Verification items for the finished model (mm, model axes). Face numbers are marked on the shaded views. A direction names the side the tool comes from. Coordinates: 2 decimals unless noted, no trailing zeros. Write each loop counter-clockwise with the first axis right and the second up, starting at its lowest first coordinate (ties: lowest second). Pieces come first, ordered by that corner, then holes. Notation, with made-up numbers: (-38, 71.25) -> (3, 71.25) arc R23 ccw to (3, 103.25) -> close; hole circle Ø6 at (33, 22). An arc over 180 degrees is marked (long way). Answer in a Markdown table with one row per item.
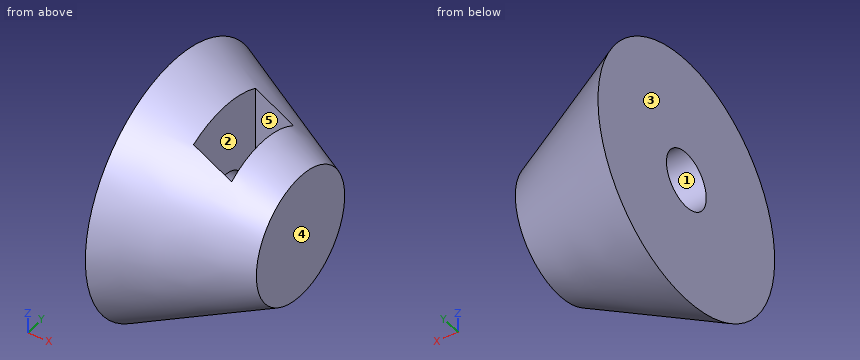
Autodesk Inventor part; units mm, degrees
ref_plane "Work Plane1" through (7, 0, 0) normal (1, 0, 0) x (0, 1, 0)
ref_plane "XZ Plane" through (0, 0, 0) normal (0, 1, 0) x (-1, 0, 0)
ref_plane "XY Plane" through (0, 0, 0) normal (0, 0, 1) x (1, 0, 0)
ref_plane "Work Plane1" through (7, 0, 0) normal (1, 0, 0) x (0, 1, 0)
sketch "Sketch1" plane through (0, 0, 0) normal (0, 1, 0) x (-1, 0, 0)
  line L0 (0, 0) -> (-10, 0)
  line L1 (0, 0) -> (0, -10)
  line L2 (-10, 0) -> (-10, -5)
  line L3 (-10, -5) -> (0, -10)
  dimension "d0" = 10
  dimension "d1" = 10
  dimension "d2" = 5
revolve "Revolution1" add sketch "Sketch1" angle 360 about axis through (0, 0, 0) along (1, 0, 0)
sketch "Sketch2" plane through (7, 0, 0) normal (1, 0, 0) x (0, 1, 0)
  circle A0 centre (0, 0) radius 2.25
  dimension "d5" = 4.5
extrude "Extrusion1" cut sketch "Sketch2" along normal blind 2 and the other way blind 10
sketch "Sketch3" plane through (7, 0, 0) normal (1, 0, 0) x (0, 1, 0)
  line L0 (-3.5, 3.5) -> (3.5, 3.5)
  line L1 (3.5, 3.5) -> (3.5, -3.5)
  line L2 (3.5, -3.5) -> (-3.5, -3.5)
  line L3 (-3.5, -3.5) -> (-3.5, 3.5)
  line L4 (-3.5, 3.5) -> (3.5, -3.5) construction
  line L5 (3.5, 3.5) -> (-3.5, -3.5) construction
  line L6 (-3.5, 3.5) -> (3.5, 3.5)
  line L7 (3.5, 3.5) -> (3.5, 13.5)
  line L8 (3.5, 13.5) -> (-3.5, 13.5)
  line L9 (-3.5, 13.5) -> (-3.5, 3.5)
  point P0 (0, 0)
  dimension "d18" = 7
  dimension "d19" = 7
  dimension "d20" = 7
  dimension "d21" = 10
extrude "Extrusion2" cut sketch "Sketch3" against normal blind 3
sketch "Sketch5" plane through (9, 0, 0) normal (-1, 0, 0) x (0, 0, 1)
  circle A0 centre (0, 0) radius 2.25
extrude "Extrusion3" add sketch "Sketch5" along normal up to surface (2 mm away)
properties part number "stollen_m4_vierkant"
1. Sectioned sample at A-A, the plane y = 0. Record the cut outline in (x, z).
Findings below:
| item | result |
|---|---|
| outline | (0, -10) -> (10, -5) -> (10, 5) -> (7, 6.5) -> (7, -3.5) -> (4, -3.5) -> (4, -2.25) -> (0, -2.25) -> close; (0, 2.25) -> (4, 2.25) -> (4, 8) -> (0, 10) -> close |
2. Access from +Z, -Z, +X, -X, +Y, -Y to the whole of each face (thin tool, end or side, straight path). Record for the marked faces 4 and 5.
Findings below:
| item | result |
|---|---|
| face 4 | +Z, -Z, +X, +Y, -Y |
| face 5 | +Z |
3. Go/stop test with flat-tipped pins: pin 1 (1 mm diameter, centred on x = 5, y = -4.5, fed in from +Z); pin 2 (2.5 mm diameter, centred on x = 5.5, y = -1.5, fed in from +Z); pin 3 (0.9 mm diameter, centred on x = 6, z = -0.5, fed in from +Y). Record where each tip stops, or that it passes through.
Findings below:
| item | result |
|---|---|
| pin 1 | stops at z = 6.46 |
| pin 2 | stops at z = -3.5 |
| pin 3 | stops at y = 7.21 |
4. Material ranges on probe 1 along X at (y, z) = (0.25, 4.75); probe 2 along X at (y, z) = (-2, 6.75); probe 3 along Z at (x, y) = (2.05, 0) (3 decimals), recorded low to high. Write a range as from..to.
Findings below:
| item | result |
|---|---|
| probe 1 | x = 0..4, 7..10 |
| probe 2 | x = 0..4 |
| probe 3 | z = -8.975..-2.25, 2.25..8.975 |
5. Release check for a two-part mould opening along X. For the marked faces 1, 2 and 3 record: released by +X, released by -X, zero draft, split by the parting line, or undercut.
Findings below:
| item | result |
|---|---|
| face 1 | zero draft |
| face 2 | undercut |
| face 3 | released by -X |
6. Sectioned sample at C-C, the plane x = 2. Record the cut outline in (y, z).
Findings below:
| item | result |
|---|---|
| outline | circle Ø18 at (0, 0); hole circle Ø4.5 at (0, 0) |
7. Sectioned sample at B-B, the plane z = 0. Record the cut outline in (x, y).
Findings below:
| item | result |
|---|---|
| outline | (0, -10) -> (10, -5) -> (10, 5) -> (0, 10) -> (0, 2.25) -> (4, 2.25) -> (4, 3.5) -> (7, 3.5) -> (7, -3.5) -> (4, -3.5) -> (4, -2.25) -> (0, -2.25) -> close |
8. Sectioned sample at D-D, the plane x = 8.5. Record the cut outline in (y, z).
Findings below:
| item | result |
|---|---|
| outline | circle Ø11.5 at (0, 0) |
